Autodesk Inventor part; units mm, degrees
ref_plane "YZ Plane" through (0, 0, 0) normal (1, 0, 0) x (0, 1, 0)
ref_plane "XZ Plane" through (0, 0, 0) normal (0, 1, 0) x (-1, 0, 0)
ref_plane "XY Plane" through (0, 0, 0) normal (0, 0, 1) x (1, 0, 0)
sketch "main" plane through (0, 0, 0) normal (0, 0, 1) x (1, 0, 0)
  arc A0 (-76.9765, 33.0075) -> (-80.2841, 30.5888) centre (-75.0825, 26.9465) ccw
  circle A1 centre (-77.4831, 23.5181) radius 2.1844
  circle A2 centre (-76.8428, -4.4337) radius 2.1844
  arc A3 (-57.2294, -80.4633) -> (-56.4581, -83.5168) centre (-56.6485, -81.9407) ccw
  circle A4 centre (-92.052, 2.7116) radius 2.1844
  circle A5 centre (-78.8735, -14.4473) radius 5.5563
  line L0 (-80.2841, 30.5888) -> (-98.7239, 4.254)
  arc A6 (-98.7239, 4.254) -> (-98.6909, -3.0772) centre (-93.5223, 0.6117) ccw
  arc A7 (-86.6264, -19.9807) -> (-70.0421, -18.0155) centre (-78.8735, -14.4473) ccw
  line L1 (-98.6909, -3.0772) -> (-86.6264, -19.9807)
  arc A8 (87.0859, 64.3881) -> (80.3336, 82.1644) centre (83.1745, 73.0729) ccw
  line L2 (86.3241, 76.2225) -> (80.0249, 76.2225)
  line L3 (80.0249, 76.2225) -> (80.0249, 69.9233)
  line L4 (80.0249, 69.9233) -> (86.3241, 69.9233)
  line L5 (86.3241, 69.9233) -> (86.3241, 76.2225)
  line L6 (86.3241, 76.2225) -> (80.0249, 69.9233) construction
  line L7 (80.0249, 76.2225) -> (86.3241, 69.9233) construction
  circle A9 centre (60.3149, 62.0006) radius 2.1844
  line L8 (87.0859, 64.3881) -> (-50.3044, 2.5112)
  arc A10 (-50.3044, 2.5112) -> (-70.0421, -18.0155) centre (-34.6127, -32.3302) ccw
  line L9 (80.3336, 82.1644) -> (-76.9765, 33.0075)
  point P0 (-51.4681, 8.9463)
  point P1 (-79.4455, 31.7864)
  point P2 (-101.2988, 0.5767)
  dimension "d4" = 11.1125
  dimension "d5" = 19.05
  dimension "d6" = 19.05
  dimension "d7" = 38.1
  dimension "d8" = 4.3688
  dimension "d9" = 6.35
  dimension "d10" = 25.4
  dimension "d11" = 6.35
  dimension "d13" = 4.3688
  dimension "d20" = 6.2992
  dimension "d21" = 6.2992
  dimension "d24" = 4.3688
  dimension "d25" = 25.4
sketch "Sketch1" plane through (0, 0, 0) normal (0, 1, 0) x (-1, 0, 0)
  arc A0 (-160.151, -40.0654) -> (-163.4586, -42.4842) centre (-158.257, -46.1264) ccw
  circle A1 centre (-160.6577, -49.5549) radius 2.1844
  circle A2 centre (-160.0174, -77.5067) radius 2.1844
  arc A3 (-140.4039, -153.5363) -> (-139.6326, -156.5897) centre (-139.823, -155.0137) ccw
  circle A4 centre (-175.2265, -70.3613) radius 2.1844
  circle A5 centre (-162.048, -87.5202) radius 5.5563
  line L0 (-163.4586, -42.4842) -> (-181.8985, -68.819)
  arc A6 (-181.8985, -68.819) -> (-181.8654, -76.1501) centre (-176.6968, -72.4612) ccw
  arc A7 (-169.8009, -93.0537) -> (-153.2166, -91.0884) centre (-162.048, -87.5202) ccw
  line L1 (-181.8654, -76.1501) -> (-169.8009, -93.0537)
  arc A8 (3.9114, -8.6848) -> (-2.8409, 9.0915) centre (0, 0) ccw
  line L2 (3.1496, 3.1496) -> (-3.1496, 3.1496)
  line L3 (-3.1496, 3.1496) -> (-3.1496, -3.1496)
  line L4 (-3.1496, -3.1496) -> (3.1496, -3.1496)
  line L5 (3.1496, -3.1496) -> (3.1496, 3.1496)
  line L6 (3.1496, 3.1496) -> (-3.1496, -3.1496) construction
  line L7 (-3.1496, 3.1496) -> (3.1496, -3.1496) construction
  circle A9 centre (-22.8596, -11.0724) radius 2.1844
  line L8 (3.9114, -8.6848) -> (-133.4789, -70.5617)
  arc A10 (-133.4789, -70.5617) -> (-153.2166, -91.0884) centre (-117.7873, -105.4032) ccw
  line L9 (-2.8409, 9.0915) -> (-160.151, -40.0654)
  point P0 (0, 0)
extrude "Extrusion1" add sketch "Sketch1" along normal blind 1.5875
properties part number "Gusset" material "Acetal Resin, White"
Part model, mm, in its own coordinate system. Round coordinates to 2 decimals unless told otherwise and drop trailing zeros. Loops run counter-clockwise (first coordinate to the right, second up) from the corner with the lowest first, then second, coordinate; pieces in that order, holes last. Notation, with made-up numbers: (24, 15) - (68, 15) arc R12 cw to (68, 36) - close; hole circle Ø11 at (59, 80.25). An arc over 180 degrees is marked (long way). Answer as a JSON object with one key per item and string values.
Item 1: Pull direction X, two halves, no side cores. Call faces 1 (the face through (161.63, 0.78, -78.98)), 2 (the face through (175.92, 0.78, -84.48)), 3 (the face through (145.473, 0.783, -79.065)): pulls with the +X half, pulls with the -X half, needs draft (parallel to the pull), parting line crosses it, or undercut.
Output:
{"face 1": "undercut", "face 2": "pulls with the +X half", "face 3": "pulls with the -X half"}
Item 2: Band-saw the part on A-A on y = 0.35. List the corners of the cut face in (x, z) (1 decimal).
Output:
{"outline": "(-3.9, -8.7) - (133.5, -70.6) arc R38.2 cw to (153.2, -91.1) arc R9.5 ccw to (169.8, -93.1) - (181.9, -76.2) arc R6.3 ccw to (181.9, -68.8) - (163.5, -42.5) arc R6.3 ccw to (160.2, -40.1) - (2.8, 9.1) arc R9.5 ccw to start; hole (-3.1, -3.1) - (3.1, -3.1) - (3.1, 3.1) - (-3.1, 3.1) - close; hole circle Ø4.4 at (22.9, -11.1); hole circle Ø11.1 at (162, -87.5); hole circle Ø4.4 at (160, -77.5); hole circle Ø4.4 at (160.7, -49.6); hole circle Ø4.4 at (175.2, -70.4)"}
Item 3: Band-saw the part on B-B on x = 35.5. List the corners of the cut face in (y, z), plus the area to 3 significant figures.
Output:
{"outline": "(0, -26.43) - (1.59, -26.43) - (1.59, -1.11) - (0, -1.11) - close", "area": "40.2 mm2"}
Item 4: Wall check: L1, parallel to X at y = 0.7, z = -48.5; L2, parallel to X at y = 1.25, z = -90; L3, parallel to Z at x = 25.5, y = 0.1. Give the ranges that are in metal, low to high.
Output:
{"L1": "84.49 to 158.74, 162.57 to 167.67", "L2": "152.76 to 157.08, 167.02 to 171.98", "L3": "-21.93 to 2.01"}
Item 5: Pin check, flat tip, straight feed: pin 1 (2.5 mm diameter, centred on x = 160.02, z = -77.51, fed in from -Y). Stop position of the tip, or through.
Output:
{"pin 1": "through"}
Item 6: Band-saw the part on C-C on z = -29. List the corners of the cut face in (x, y), plus the area to 3 significant figures.
Output:
{"outline": "(41.2, 0) - (124.74, 0) - (124.74, 1.59) - (41.2, 1.59) - close", "area": "133 mm2"}
